Geometry: see drawing. Coordinates: mm, zero at the bounding-box minimum. A direction names the side the tool comes from. Give positions to 0.01 mm unless a question says otherwise; leave off trailing zeros. Loops run counter-clockwise (first coordinate to the right, second up) from the corner with the lowest first, then second, coordinate; pieces in that order, holes last. Notation, with made-up numbers: M 36.5,37.25 L 78.5,37.25 A22 cw 78.5,58.25 Z; hole C 12,72.5 d7. An arc over 180 degrees is marked long. Put each result on its own line as item: value.
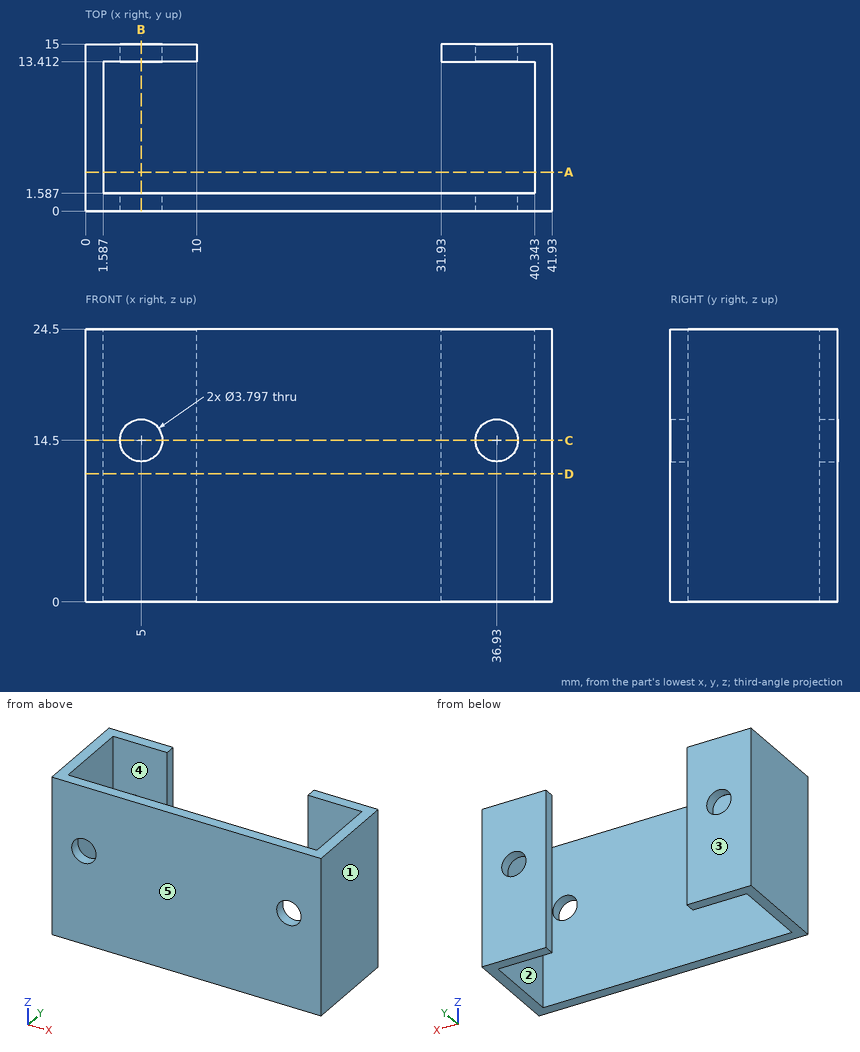
Item 1: Section C-C on z = 14.5. Output: boundary loops of the cut face in (x, y).
Output values:
outline: M 0,0 L 3.1,0 L 3.1,1.59 L 1.59,1.59 L 1.59,13.41 L 3.1,13.41 L 3.1,15 L 0,15 Z; M 6.9,0 L 35.03,0 L 35.03,1.59 L 6.9,1.59 Z; M 6.9,13.41 L 10,13.41 L 10,15 L 6.9,15 Z; M 31.93,13.41 L 35.03,13.41 L 35.03,15 L 31.93,15 Z; M 38.83,0 L 41.93,0 L 41.93,15 L 38.83,15 L 38.83,13.41 L 40.34,13.41 L 40.34,1.59 L 38.83,1.59 Z
Item 2: Set-up query: the marked faces 4 and 5. Return all of +Z, -Z, +X, -X, +Y, -Y with unobstructed straight access to the full face (end or side cutting, diameter ignored); none if empty.
Output values:
face 4: +Z, -Z
face 5: +Z, -Z, +X, -X, -Y
Item 3: Section A-A on y = 3.5. Output: boundary loops of the cut face in (x, z).
Output values:
outline: M 0,0 L 1.59,0 L 1.59,24.5 L 0,24.5 Z; M 40.34,0 L 41.93,0 L 41.93,24.5 L 40.34,24.5 Z
Item 4: Line query: probe 1 along X at (y, z) = (11, 6); probe 2 along Y at (x, z) = (32, 15); probe 3 along Z at (x, y) = (36.93, 14.55). Output: solid intervals per line, ascending. Write a range as [from, to].
Output values:
probe 1: [0, 1.59], [40.34, 41.93]
probe 2: [0, 1.59], [13.41, 15]
probe 3: [0, 12.6], [16.4, 24.5]
Item 5: Section B-B on x = 5. Output: boundary loops of the cut face in (y, z).
Output values:
outline: M 0,0 L 1.59,0 L 1.59,12.6 L 0,12.6 Z; M 0,16.4 L 1.59,16.4 L 1.59,24.5 L 0,24.5 Z; M 13.41,0 L 15,0 L 15,12.6 L 13.41,12.6 Z; M 13.41,16.4 L 15,16.4 L 15,24.5 L 13.41,24.5 Z
Item 6: Section D-D on z = 11.5. Output: boundary loops of the cut face in (x, y), then the cut area to 3 significant figures.
Output values:
outline: M 0,0 L 41.93,0 L 41.93,15 L 31.93,15 L 31.93,13.41 L 40.34,13.41 L 40.34,1.59 L 1.59,1.59 L 1.59,13.41 L 10,13.41 L 10,15 L 0,15 Z
area: 136 mm²
Item 7: Pin query (flat end, axial travel): pin 1 Ø2.5 at (x, z) = (35, 9.5) entering from -Y; pin 2 Ø3.5 at (x, z) = (36.93, 14.5) entering from +Y; pin 3 Ø10 at (x, z) = (22.5, 6) entering from +Y. Return the tip coordinate at first contact, or that it passes through.
Output values:
pin 1: y = 0
pin 2: through
pin 3: y = 1.59
Item 8: Mould query, pull axis Y, two halves, no side actions, for the marked faces 1, 2 and 3. Classes: pulls with the +Y half, pulls with the -Y half, needs draft (parallel to the pull), parting line crosses it, or undercut.
Output values:
face 1: needs draft
face 2: undercut
face 3: pulls with the +Y half
